Part print with two shaded views. Sizes in mm from the minimum x, y, z corner. A direction names the side the tool comes from. Round coordinates to 2 decimals unless told otherwise and drop trailing zeros. Write each loop counter-clockwise with the first axis right and the second up, starting at its lowest first coordinate (ties: lowest second). Pieces come first, ordered by that corner, then holes. Notation, with made-up numbers: (-13.75, 82.25) - (-9.75, 82.25) arc R24 ccw to (-9.75, 98.25) - close; hole circle Ø9 at (31.5, -31.75). An arc over 180 degrees is marked (long way). Answer as a JSON object with one key per item and string values. Group by question number.
Item 1: Flat gauge pins, fed straight in: pin 1 (2 mm diameter, centred on x = 5, y = 1.5, fed in from +Z); pin 2 (3 mm diameter, centred on y = 7, z = 8.5, fed in from -X); pin 3 (2 mm diameter, centred on x = 7.5, z = 11, fed in from +Y). Where does each tip first touch, or does it go through?
Item 2: Probe line 1 (Y direction, x = 12.25, z = 8); line 2 (X direction, y = 2.25, z = 5); line 3 (Z direction, x = 12.5, y = 8.25). List the from-to ranges inside material, lowest first. Write a range as from..to.
Item 3: Slice it at C-C, the plane y = 7. List the corners of the cut face in (x, z), then the cut area to 3 significant figures.
Item 4: Which spindle directions (+Z, -Z, +X, -X, +Y, -Y) get a long thin tool onto all of the face, cutting with end or side? Do the marked faces 1 and 2. Say none if no direction does.
Item 5: Slice it at A-A, the plane x = 5. List the corners of the cut face in (y, z), then the cut area to 3 significant figures.
Item 6: Slice it at B-B, the plane z = 8. List the corners of the cut face in (x, y), then the cut area to 3 significant figures.
Item 7: Two-plate mould, pull along Z, no slides. Class the marked faces 3, 4 and 5: +Z half, -Z half, draft (parallel to the pull), parting line (faces both ways), or undercut.
Item 8: Slice it at D-D, the plane z = 1. List the corners of the cut face in (x, y).
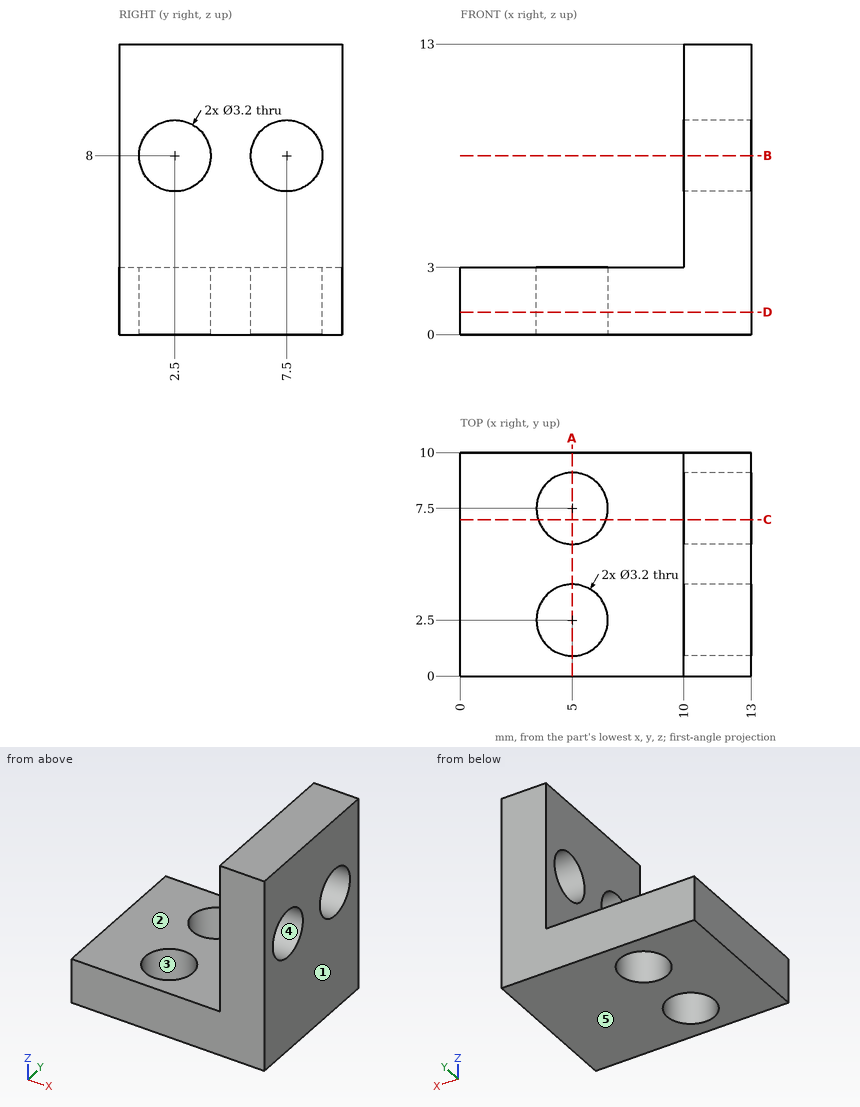
Geometry says:
{
 "1": {"pin 1": "stops at z = 3", "pin 2": "stops at x = 10", "pin 3": "passes through"},
 "2": {"line 1": "y = 0..0.9, 4.1..5.9, 9.1..10", "line 2": "x = 10..13", "line 3": "z = 0..6.59, 9.41..13"},
 "3": {"outline": "(0, 0) - (3.48, 0) - (3.48, 3) - (0, 3) - close; (6.52, 0) - (13, 0) - (13, 6.48) - (10, 6.48) - (10, 3) - (6.52, 3) - close; (10, 9.52) - (13, 9.52) - (13, 13) - (10, 13) - close", "area": "50.8 mm^2"},
 "4": {"face 1": "+Z, -Z, +X, +Y, -Y", "face 2": "+Z, -X, +Y, -Y"},
 "5": {"outline": "(0, 0) - (0.9, 0) - (0.9, 3) - (0, 3) - close; (4.1, 0) - (5.9, 0) - (5.9, 3) - (4.1, 3) - close; (9.1, 0) - (10, 0) - (10, 3) - (9.1, 3) - close", "area": "10.8 mm^2"},
 "6": {"outline": "(10, 0) - (13, 0) - (13, 0.9) - (10, 0.9) - close; (10, 4.1) - (13, 4.1) - (13, 5.9) - (10, 5.9) - close; (10, 9.1) - (13, 9.1) - (13, 10) - (10, 10) - close", "area": "10.8 mm^2"},
 "7": {"face 3": "draft", "face 4": "undercut", "face 5": "-Z half"},
 "8": {"outline": "(0, 0) - (13, 0) - (13, 10) - (0, 10) - close; hole circle Ø3.2 at (5, 2.5); hole circle Ø3.2 at (5, 7.5)"}
}
